Verification items for the finished model (mm, model axes). Face numbers are marked on the shaded views. A direction names the side the tool comes from. Round coordinates to 2 decimals unless told otherwise and drop trailing zeros. Loops run counter-clockwise (first coordinate to the right, second up) from the corner with the lowest first, then second, coordinate; pieces in that order, holes last. Notation, with made-up numbers: (24, -21.5) - (68, -21.5) arc R20 ccw to (68, -5.5) - close; hole circle Ø9 at (83.25, 56). An arc over 180 degrees is marked (long way). Use CSV: the item, a comma, the result in double quotes.
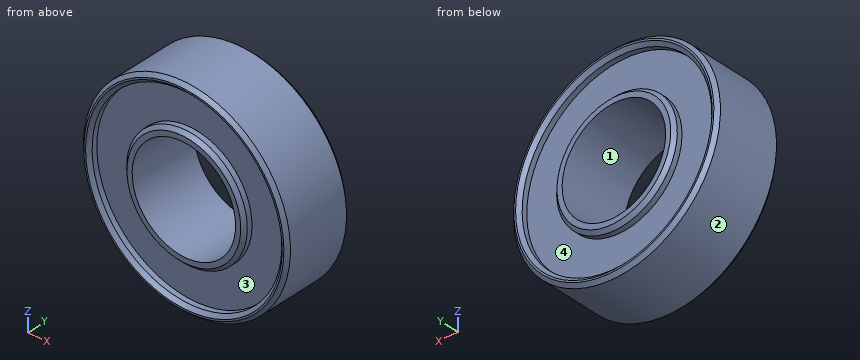
```python
from build123d import *

# Parameters (mm, degrees)
SKETCH_1_R          = 3
EXTRUDE_1_DEPTH     = 2
SKETCH_2_R          = 1.5
CUT_EXTRUDE_1_DEPTH = 2
CUT_EXTRUDE_START   = 2
SKETCH_3_R          = 2.75
SKETCH_3_R_2        = 1.75
CUT_EXTRUDE_2_DEPTH = 0.25
CUT_EXTRUDE_START_2 = 0.25
SKETCH_4_R          = 2.75
SKETCH_4_R_2        = 1.75
CUT_EXTRUDE_3_DEPTH = 0.25
CHAMFER_1_SIZE      = 0.1


with BuildPart() as part:
    # 草图1 → 凸台-拉伸1 (new body)
    with BuildSketch(Plane(origin=(0, 0, 0), x_dir=(1, 0, 0), z_dir=(0, 1, 0))):
        with Locations(Location((0, 0, 0), (0, 0, 270))):
            Circle(SKETCH_1_R)
    extrude(amount=EXTRUDE_1_DEPTH)

    # 草图2 → 切除-拉伸1 (cut)
    with BuildSketch(Plane(origin=(0, 0, 0), x_dir=(1, 0, 0), z_dir=(0, 1, 0))):
        with Locations(Location((0, 0, 0), (0, 0, 270))):
            Circle(SKETCH_2_R)
    extrude(amount=CUT_EXTRUDE_1_DEPTH, mode=Mode.SUBTRACT)

    # 草图3 → 切除-拉伸2 (cut)
    with BuildSketch(Plane(origin=(0, 0, 0), x_dir=(1, 0, 0), z_dir=(0, 1, 0)).offset(CUT_EXTRUDE_START)):
        with Locations(Location((0, 0, 0), (0, 0, 270))):
            Circle(SKETCH_3_R)
        with Locations(Location((0, 0, 0), (0, 0, 270))):
            Circle(SKETCH_3_R_2, mode=Mode.SUBTRACT)
    extrude(amount=-CUT_EXTRUDE_2_DEPTH, mode=Mode.SUBTRACT)

    # 草图4 → 切除-拉伸3 (cut)
    with BuildSketch(Plane(origin=(0, 0, 0), x_dir=(1, 0, 0), z_dir=(0, 1, 0)).offset(CUT_EXTRUDE_START_2)):
        with Locations(Location((0, 0, 0), (0, 0, 270))):
            Circle(SKETCH_4_R)
        with Locations(Location((0, 0, 0), (0, 0, 270))):
            Circle(SKETCH_4_R_2, mode=Mode.SUBTRACT)
    extrude(amount=-CUT_EXTRUDE_3_DEPTH, mode=Mode.SUBTRACT)

    # 倒角1
    chamfer_1_edges = [part.edges().sort_by_distance(p)[0] for p in [
        (0, 2, -2.75),
        (0, 2, -1.75),
        (0, 0, -1.75),
        (0, 0, -2.75),
        (0, 0, -3),
        (0, 2, -3),
    ]]
    chamfer(chamfer_1_edges, length=CHAMFER_1_SIZE)


solid = part.part
```
1) Access from +Z, -Z, +X, -X, +Y, -Y to the whole of each face (thin tool, end or side, straight path). Record for the marked faces 3 and 4.
Returned:
face 3,"-Y"
face 4,"+Y"
2) Mould release check, pull along X, two halves, no side actions. Record for the marked faces 1 and 2: +X half, -X half, draft (parallel to the pull), parting line (faces both ways), or undercut.
Returned:
face 1,"undercut"
face 2,"parting line"
3) Gauge pin test, flat ends, axial feed: pin 1 Ø1 at (y, z) = (1.5, -1.5) entering from +X; pin 2 Ø1.8 at (x, z) = (0, 0) entering from +Y; pin 3 Ø1 at (x, y) = (1, 1.5) entering from +Z. Record the tip position at first contact, or that the pin passes through.
Returned:
pin 1,"stops at x = 2.83"
pin 2,"passes through"
pin 3,"stops at z = 2.96"
4) Cross-section at A-A, the plane y = 0.4. Record the cut outline in (x, z).
Returned:
outline,"circle Ø6 at (0, 0); hole circle Ø3 at (0, 0)"
5) Thickness scan on probe 1 along X at (y, z) = (0.2, 0); probe 2 along X at (y, z) = (0.2, -1.15); probe 3 along X at (y, z) = (1.6, 0). Record the ranges inside material, lowest first. Write a range as [from, to].
Returned:
probe 1,"x = [-3, -2.75], [-1.75, -1.5], [1.5, 1.75], [2.75, 3]"
probe 2,"x = [-2.77, -2.5], [-1.32, -0.96], [0.96, 1.32], [2.5, 2.77]"
probe 3,"x = [-3, -1.5], [1.5, 3]"
